Geometry check sheet. Reference: the model listing, model coordinates, mm. Face numbers are marked on the shaded views. A direction names the side the tool comes from. Give positions to 0.01 mm unless a question says otherwise; leave off trailing zeros. Loops run counter-clockwise (first coordinate to the right, second up) from the corner with the lowest first, then second, coordinate; pieces in that order, holes last. Notation, with made-up numbers: (21, 4.5) - (60, 4.5) arc R24 ccw to (60, 34.5) - close; hole circle Ø7 at (21, 36.25). An arc over 180 degrees is marked (long way). Write item = value, one per line. Start each with the question number.
from build123d import *

# Parameters (mm, degrees)
F1_DEPTH = 609.092
F3_W     = 76.98
F3_H     = 338.836
F3_W_2   = 46.863
F4_DEPTH = 25.4
F6_R     = 15.875
F7_DEPTH = 25.4
F8_D     = 7.14375


# Not quite as in the source:
# - a length typed as a fraction of an inch, garbled in the dataset ("3 / 203.2 mm" for 3/8 in), is restored


with BuildPart() as f1:
    # F0 (on Front) → F1 (new body)
    with BuildSketch(Plane.XZ):
        Polygon((0, -3.175), (0, 0), (-26.162, 0), (-26.162, 126.873), (-499.364, 126.873), (-499.364, 0), (-525.272, 0), (-525.272, -3.175), (-496.189, -3.175), (-496.189, 123.698), (-29.337, 123.698), (-29.337, -3.175), align=None)
    extrude(amount=F1_DEPTH)

    # F3 (on face) → F4 (cut)
    with BuildSketch(Plane.XY.offset(126.873)):
        with Locations((-390.262, -241.3)):
            Rectangle(F3_W, F3_H)
        with Locations((-255.262, -241.3)):
            Rectangle(F3_W_2, F3_H)
    extrude(amount=-F4_DEPTH, mode=Mode.SUBTRACT)

    # F6 (on face) → F7 (cut)
    with BuildSketch(Plane.XY.offset(126.873)):
        with Locations((-418.846, -544.068)):
            Circle(F6_R)
    extrude(amount=-F7_DEPTH, mode=Mode.SUBTRACT)

    # F8 (through all)
    with Locations(Plane.XY):
        with Locations((-512.318, -25.908), (-512.318, -212.09), (-512.318, -397.002), (-512.318, -582.93), (-12.954, -582.93), (-12.954, -397.002), (-12.954, -212.09), (-12.954, -25.908)):
            Hole(F8_D / 2)


solid = f1.part
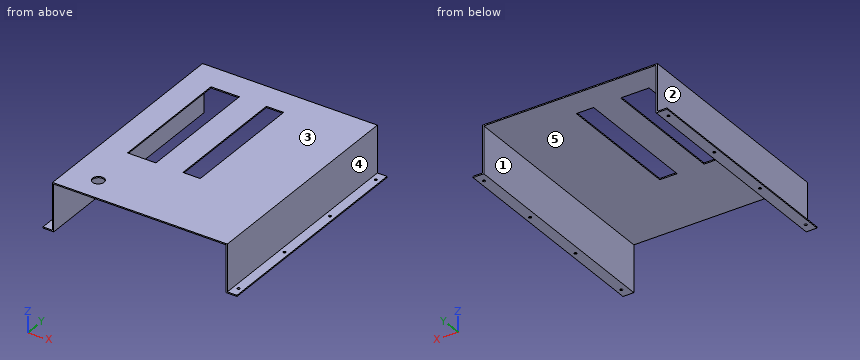
1) Release check for a two-part mould opening along X. For the marked faces 3, 4 and 5 record: pulls with the +X half, pulls with the -X half, needs draft (parallel to the pull), parting line crosses it, or undercut.
2) Cross-section at B-B on z = 64.5. Enter the section's corners in (x, y), and give its area (3 significant figures).
3) Tool access check on the marked faces 1 and 2. Record the directions out of +Z, -Z, +X, -X, +Y, -Y that give a thin tool (end or side, any length) a straight path to the whole face; none if there is none.
4) Material ranges on line 1 along X through (y, z) = (-212, -2); line 2 along X through (y, z) = (-402, 20); line 3 along Z through (x, y) = (-304, -375), recorded low to high.
5) Cross-section at A-A on x = -241.5. Enter the section's corners in (y, z).
6) Cross-section at D-D on x = -480. Enter the section's corners in (y, z), and give its area (3 significant figures).
7) Cross-section at C-C on y = -130. Enter the section's corners in (x, z) (1 decimal), and give its area (3 significant figures).
8) Gauge pin test, flat ends, axial feed: P1, Ø20.5, axis at x = -518.5, y = -350, coming from the +Z side; P2, Ø8, axis at x = -12.954, y = -212.09, coming from the -Z side (3 decimals); P3, Ø1, axis at y = -299, z = 125, coming from the +X side; P4, Ø4, axis at y = -403.5, z = 33.5, coming from the -X side. Record the tip position at first contact, or that the pin passes through.
Checked values:
q1.face_3 = needs draft
q1.face_4 = pulls with the +X half
q1.face_5 = undercut
q2.outline = (-499.36, -609.09) - (-496.19, -609.09) - (-496.19, 0) - (-499.36, 0) - close; (-29.34, -609.09) - (-26.16, -609.09) - (-26.16, 0) - (-29.34, 0) - close
q2.area = 3,870 mm²
q3.face_1 = -Z, +Y, -Y
q3.face_2 = +Z, -X, +Y, -Y
q4.line_1 = -525.27 to -515.89, -508.75 to -496.19, -29.34 to -16.52, -9.38 to 0
q4.line_2 = -499.36 to -496.19, -29.34 to -26.16
q4.line_3 = 123.7 to 126.87
q5.outline = (-609.09, 123.7) - (-410.72, 123.7) - (-410.72, 126.87) - (-609.09, 126.87) - close; (-71.88, 123.7) - (0, 123.7) - (0, 126.87) - (-71.88, 126.87) - close
q6.outline = (-609.09, 123.7) - (0, 123.7) - (0, 126.87) - (-609.09, 126.87) - close
q6.area = 1,930 mm²
q7.outline = (-525.3, -3.2) - (-496.2, -3.2) - (-496.2, 123.7) - (-428.8, 123.7) - (-428.8, 126.9) - (-499.4, 126.9) - (-499.4, 0) - (-525.3, 0) - close; (-351.8, 123.7) - (-278.7, 123.7) - (-278.7, 126.9) - (-351.8, 126.9) - close; (-231.8, 123.7) - (-29.3, 123.7) - (-29.3, -3.2) - (0, -3.2) - (0, 0) - (-26.2, 0) - (-26.2, 126.9) - (-231.8, 126.9) - close
q7.area = 2,080 mm²
q8.P1 = 0
q8.P2 = -3.175
q8.P3 = -26.16
q8.P4 = -499.36
